Verification items for the finished model (mm, model axes). A direction names the side the tool comes from. Coordinates: 2 decimals unless noted, no trailing zeros. Write each loop counter-clockwise with the first axis right and the second up, starting at its lowest first coordinate (ties: lowest second). Pieces come first, ordered by that corner, then holes. Notation, with made-up numbers: (-18.75, 27) -> (-0.75, 27) arc R20 ccw to (-0.75, 58) -> close; hole circle Ø2 at (70.25, 50). An arc over 180 degrees is marked (long way). Answer in a Markdown table with one row per item.
```python
from build123d import *

# Parameters (mm, degrees)
F0_R     = 45
F0_R_2   = 30
F0_R_3   = 20
F1_DEPTH = 90
F2_DEPTH = 70
F3_DEPTH = 40
F5_DEPTH = 50
F4_R     = 15
F6_DEPTH = 50
F8_DEPTH = 50
F10_D    = 20


with BuildPart() as f1:
    # F0 (on Top) → F1 (new body)
    with BuildSketch(Plane.XY):
        Circle(F0_R)
        Circle(F0_R_2, mode=Mode.SUBTRACT)
        Circle(F0_R_2)
        Circle(F0_R_3, mode=Mode.SUBTRACT)
        Circle(F0_R_3)
    extrude(amount=F1_DEPTH)

    # F0 (on Top) → F2 (join)
    with BuildSketch(Plane.XY):
        Circle(F0_R_3)
    extrude(amount=-F2_DEPTH)

    # F0 (on Top) → F3 (join)
    with BuildSketch(Plane.XY):
        Circle(F0_R_2)
        Circle(F0_R_3, mode=Mode.SUBTRACT)
    extrude(amount=-F3_DEPTH)

    # F4 (on Right) → F5 (cut, symmetric)
    with BuildSketch(Plane.YZ):
        with BuildLine():
            Line((-82.7872549732, 115.9372627735), (-82.7872549732, 30))
            Line((-82.7872549732, 30), (-40, 30))
            ThreePointArc((-40, 30), (-32.9289321881, 32.9289321881), (-30, 40))
            Line((-30, 40), (-30, 60))
            ThreePointArc((-30, 60), (0, 90), (30, 60))
            Line((30, 60), (30, 40))
            ThreePointArc((30, 40), (32.9289321881, 32.9289321881), (40, 30))
            Line((40, 30), (82.7872549732, 30))
            Line((82.7872549732, 30), (82.7872549732, 115.9372627735))
            Line((82.7872549732, 115.9372627735), (-82.7872549732, 115.9372627735))
        make_face()
    extrude(amount=F5_DEPTH, both=True, mode=Mode.SUBTRACT)

    # F4 (on Right) → F6 (cut, symmetric)
    with BuildSketch(Plane.YZ):
        with Locations((0, 60)):
            Circle(F4_R)
    extrude(amount=F6_DEPTH, both=True, mode=Mode.SUBTRACT)

    # F7 (on Front) → F8 (cut, symmetric)
    with BuildSketch(Plane.XZ):
        with BuildLine():
            Line((20, 128.1329473248), (-20, 128.1329473248))
            Line((-20, 128.1329473248), (-20, 40))
            ThreePointArc((-20, 40), (-17.0710678119, 32.9289321881), (-10, 30))
            Line((-10, 30), (10, 30))
            ThreePointArc((10, 30), (17.0710678119, 32.9289321881), (20, 40))
            Line((20, 40), (20, 128.1329473248))
        make_face()
    extrude(amount=F8_DEPTH, both=True, mode=Mode.SUBTRACT)

    # F10 (through all)
    with Locations(Plane(origin=(0, 0, -70), x_dir=(1, 0, 0), z_dir=(0, 0, -1))):
        with Locations((0, 0)):
            Hole(F10_D / 2)


solid = f1.part
```
1. Tool access check on faces 1 (the flat face through (-27, 30, 50)), 2 (the cylindrical face through (32.675, 13.856, 54.255)), 3 (the cylindrical face through (-4.336, -19.524, -54.79)). Record the directions out of +Z, -Z, +X, -X, +Y, -Y that give a thin tool (end or side, any length) a straight path to the whole face; none if there is none.
Geometry says:
| item | result |
|---|---|
| face 1 | +Z, +X, -X, +Y |
| face 2 | +X, -X |
| face 3 | -Z |
2. Section check C-C, the plane z = -34.5. Record the boundary of the cut face in (x, y).
Geometry says:
| item | result |
|---|---|
| outline | circle Ø60 at (0, 0); hole circle Ø20 at (0, 0) |
3. Thickness scan on line 1 (Y direction, x = 0, z = -11); line 2 (Y direction, x = 0, z = -47); line 3 (Z direction, x = 30.75, y = 0). Record the ranges inside material, lowest first. Write a range as from..to.
Geometry says:
| item | result |
|---|---|
| line 1 | -30..-10, 10..30 |
| line 2 | -20..-10, 10..20 |
| line 3 | 0..45, 75..90 |
4. Section check D-D, the plane x = -39. Record the boundary of the cut face in (y, z).
Geometry says:
| item | result |
|---|---|
| outline | (-22.45, 0) -> (22.45, 0) -> (22.45, 79.9) arc R30 ccw to (-22.45, 79.9) -> close; hole circle Ø30 at (0, 60) |
5. Section check A-A, the plane x = 5.5. Record the boundary of the cut face in (y, z), plus the area to 3 significant figures.
Geometry says:
| item | result |
|---|---|
| outline | (-44.66, 0) -> (-29.49, 0) -> (-29.49, -40) -> (-19.23, -40) -> (-19.23, -70) -> (-8.35, -70) -> (-8.35, 30) -> (-44.66, 30) -> close; (8.35, -70) -> (19.23, -70) -> (19.23, -40) -> (29.49, -40) -> (29.49, 0) -> (44.66, 0) -> (44.66, 30) -> (8.35, 30) -> close |
| area | 4,520 mm^2 |
6. Depth check by flat-ended pin: P1, Ø15, axis at x = -25.5, z = 52.5, coming from the -Y side; P2, Ø23, axis at x = 0, y = 0, coming from the +Z side; P3, Ø4, axis at x = 29, z = 50, coming from the +Y side. Enter the tip coordinate at first touch or a pass-through.
Geometry says:
| item | result |
|---|---|
| P1 | y = -30 |
| P2 | z = 30.11 |
| P3 | y = 30 |
7. Section check B-B, the plane y = -4. State how many separate pieces and enclosed holes the cut face has, plus the area to 3 significant figures.
Geometry says:
| item | result |
|---|---|
| separate pieces | 4 |
| enclosed holes | 0 |
| area | 5,980 mm^2 |
8. Mould release check, pull along X, two halves, no side actions. Record for faces 4 (the flat face through (27, 30, 50)), 5 (the flat face through (20, 0, 76)), 6 (the cylindrical face through (-29.97, 1.32, -19.72)): released by +X, released by -X, zero draft, split by the parting line, or undercut.
Geometry says:
| item | result |
|---|---|
| face 4 | zero draft |
| face 5 | undercut |
| face 6 | split by the parting line |
